Geometry: final body of the model. Coordinates: model frame, mm. Face numbers are marked on the shaded views. A direction names the side the tool comes from. Give positions to 0.01 mm unless a question says otherwise; leave off trailing zeros. Loops run counter-clockwise (first coordinate to the right, second up) from the corner with the lowest first, then second, coordinate; pieces in that order, holes last. Notation, with made-up numbers: (56, 80.25) -> (95, 80.25) arc R15 ccw to (95, 84.25) -> close; hole circle Ø5 at (65.25, -33.75). An arc over 180 degrees is marked (long way). Answer in a Markdown table with one row per item. Add a question column.
1) First-contact query: P1, Ø2, axis at x = -13, z = 0, coming from the +Y side; P2, Ø10, axis at x = 9.5, y = 82.5, coming from the +Z side; P3, Ø8, axis at y = 36, z = 14, coming from the +X side. Flat tips, straight axial feed; report the tip coordinate or a pass-through.
2) Line query: line 1 (Y direction, x = -3.5, z = -10); line 2 (X direction, y = 83.6, z = -13); line 3 (Y direction, x = 1, z = -4). Output: solid intervals per line, ascending. Write a range as from..to.
3) Section query A-A (y = 83.5). Return the cut outline in (x, z).
4) Access query for the marked faces 1, 2, 3 and 4. Directions: +Z, -Z, +X, -X, +Y, -Y. A direction counts if a zero-diameter tool reaches every point of the face in a straight line with its end or side. Return the directions, or none.
5) Section query D-D (y = 38). Return the cut outline in (x, z), plus the area to 3 significant figures.
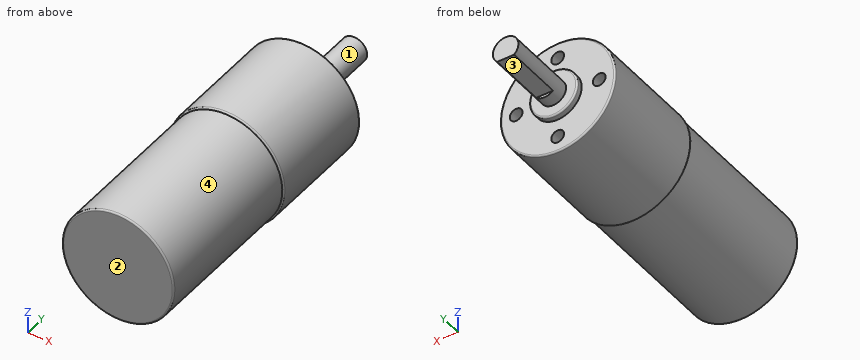
```python
from build123d import *

# Parameters (mm, degrees)
SKETCH_1_R          = 17.5
EXTRUDE_1_DEPTH     = 50
SKETCH_3_R          = 18
EXTRUDE_4_DEPTH     = 35
SKETCH_4_R          = 7.5
EXTRUDE_5_DEPTH     = 2
SKETCH_5_R          = 4
EXTRUDE_6_DEPTH     = 22
SKETCH_6_R          = 2
CUT_EXTRUDE_1_DEPTH = 5
SKETCH_7_W          = 8.061647896
SKETCH_7_H          = 1.71902786
CUT_EXTRUDE_2_DEPTH = 18
FILLET_10_R         = 0.5
FILLET_11_R         = 0.5
FILLET_12_R         = 0.5
FILLET_13_R         = 0.5


with BuildPart() as part:
    # 草图1 → 凸台-拉伸1 (new body)
    with BuildSketch(Plane(origin=(0, 0, 0), x_dir=(1, 0, 0), z_dir=(0, 1, 0))):
        with Locations(Location((0, 0, 0), (0, 0, 270))):
            Circle(SKETCH_1_R)
    extrude(amount=EXTRUDE_1_DEPTH)

    # 草图3 → 凸台-拉伸4 (add)
    with BuildSketch(Plane(origin=(0, 50, 0), x_dir=(1, 0, 0), z_dir=(0, 1, 0))):
        with Locations(Location((0, 0, 0), (0, 0, 270))):
            Circle(SKETCH_3_R)
    extrude(amount=EXTRUDE_4_DEPTH)

    # 草图4 → 凸台-拉伸5 (add)
    with BuildSketch(Plane(origin=(0, 85, 0), x_dir=(1, 0, 0), z_dir=(0, 1, 0))):
        with Locations(Location((0, 0, 0), (0, 0, 270))):
            Circle(SKETCH_4_R)
    extrude(amount=EXTRUDE_5_DEPTH)

    # 草图5 → 凸台-拉伸6 (add)
    with BuildSketch(Plane(origin=(0, 87, 0), x_dir=(1, 0, 0), z_dir=(0, 1, 0))):
        with Locations(Location((0, 0, 0), (0, 0, 270))):
            Circle(SKETCH_5_R)
    extrude(amount=EXTRUDE_6_DEPTH)

    # 草图6 → 切除-拉伸1 (cut)
    with BuildSketch(Plane(origin=(0, 85, 0), x_dir=(1, 0, 0), z_dir=(0, 1, 0))):
        with Locations(Location((0, 13, 0), (0, 0, 270))):
            Circle(SKETCH_6_R)
        with Locations(Location((13, 0, 0), (0, 0, 270))):
            Circle(SKETCH_6_R)
        with Locations(Location((0, -13, 0), (0, 0, 270))):
            Circle(SKETCH_6_R)
        with Locations(Location((-13, 0, 0), (0, 0, 270))):
            Circle(SKETCH_6_R)
    extrude(amount=-CUT_EXTRUDE_1_DEPTH, mode=Mode.SUBTRACT)

    # 草图7 → 切除-拉伸2 (cut)
    with BuildSketch(Plane(origin=(0, 109, 0), x_dir=(1, 0, 0), z_dir=(0, 1, 0))):
        with Locations((-0.414937759, 3.85951393)):
            Rectangle(SKETCH_7_W, SKETCH_7_H)
    extrude(amount=-CUT_EXTRUDE_2_DEPTH, mode=Mode.SUBTRACT)

    # 圆角10
    fillet_10_edges = [part.edges().sort_by_distance(p)[0] for p in [
        (0, 85, -18),
    ]]
    fillet(fillet_10_edges, radius=FILLET_10_R)

    # 圆角11
    fillet_11_edges = [part.edges().sort_by_distance(p)[0] for p in [
        (0, 50, -18),
    ]]
    fillet(fillet_11_edges, radius=FILLET_11_R - 0.0001)  # a hair under: the kernel refuses the full size

    # 圆角12
    fillet_12_edges = [part.edges().sort_by_distance(p)[0] for p in [
        (0, 0, -17.5),
    ]]
    fillet(fillet_12_edges, radius=FILLET_12_R)

    # 圆角13
    fillet_13_edges = [part.edges().sort_by_distance(p)[0] for p in [
        (0, 87, -7.5),
    ]]
    fillet(fillet_13_edges, radius=FILLET_13_R)


solid = part.part
```
Evaluation:
| question | item | result |
|---|---|---|
| 1 | P1 | y = 80 |
| 1 | P2 | z = 17.43 |
| 1 | P3 | x = 14.36 |
| 2 | line 1 | 0..85 |
| 2 | line 2 | -12.45..-2, 2..12.45 |
| 2 | line 3 | 0..87 |
| 3 | outline | circle Ø36 at (0, 0); hole circle Ø4 at (-13, 0); hole circle Ø4 at (0, -13); hole circle Ø4 at (0, 13); hole circle Ø4 at (13, 0) |
| 4 | face 1 | +Y |
| 4 | face 2 | +Z, -Z, +X, -X, -Y |
| 4 | face 3 | -Z, +X, -X, +Y |
| 4 | face 4 | -Y |
| 5 | outline | circle Ø35 at (0, 0) |
| 5 | area | 962 mm² |
